```python
from build123d import *

# Parameters (mm, degrees)
CUT_EXTRUDE1_REACH  = 125.775
SKETCH2_R           = 3.3
SKETCH3_R           = 5.5
CUT_EXTRUDE2_DEPTH  = 6
CIRPATTERN1_COUNT   = 6
BOSS_EXTRUDE1_REACH = 125.775


with BuildPart() as part:
    # Sketch1 → Revolve1 (revolve)
    with BuildSketch(Plane.XY, mode=Mode.PRIVATE) as revolve1_sk:
        Polygon((-55.75, 38), (-43.75, 38), (-43.75, 25), (5, 25), (5, 23), (7, 23), (7, 25), (55.75, 25), (55.75, 16), (-55.75, 16), align=None)
    revolve(revolve1_sk.sketch.rotate(Axis((-82.106015927, 0, 0), (1, 0, 0)), 180), axis=Axis((-82.106015927, 0, 0), (1, 0, 0)))

    # Sketch2 → Cut-Extrude1 (cut, up to next)
    with BuildSketch(Plane.ZY.offset(55.75), mode=Mode.PRIVATE) as cut_extrude1_sk1:
        with Locations(Location((0, -31.5, 0), (0, 0, 270))):
            Circle(SKETCH2_R)
    cut_extrude1_tool1 = extrude(cut_extrude1_sk1.sketch, amount=-CUT_EXTRUDE1_REACH, mode=Mode.PRIVATE) & part.part
    cut_extrude1 = cut_extrude1_tool1.solids().sort_by_distance((-55.75, -31.5, 0))[0]
    add(cut_extrude1, mode=Mode.SUBTRACT)

    # Sketch3 → Cut-Extrude2 (cut)
    with BuildSketch(Plane.ZY.offset(55.75)):
        with Locations(Location((0, -31.5, 0), (0, 0, 270))):
            Circle(SKETCH3_R)
    cut_extrude2 = extrude(amount=-CUT_EXTRUDE2_DEPTH, mode=Mode.SUBTRACT)

    # CirPattern1: Cut-Extrude1, Cut-Extrude2 ×6 about axis, 1 skipped
    cirpattern1_axis = Axis((0, 0, 0), (-1, 0, 0))
    add([cut_extrude1.rotate(cirpattern1_axis, i * 360 / CIRPATTERN1_COUNT) for i in range(1, CIRPATTERN1_COUNT) if i not in (3,)], mode=Mode.SUBTRACT)
    add([cut_extrude2.rotate(cirpattern1_axis, i * 360 / CIRPATTERN1_COUNT) for i in range(1, CIRPATTERN1_COUNT) if i not in (3,)], mode=Mode.SUBTRACT)

    # Boss-Extrude1: up to this face of the body (flat: up to its plane)
    boss_extrude1_end = Plane(part.part.faces().sort_by_distance((-43.75, 36.925197693, 0))[0])
    # Sketch5 → Boss-Extrude1 (add, up to the picked face)
    with BuildSketch(Plane(origin=(55.75, 0, 0), x_dir=(0, 0, -1), z_dir=(1, 0, 0)), mode=Mode.PRIVATE) as boss_extrude1_sk1:
        with BuildLine():
            Line((-19, 30), (19, 30))
            Line((19, 30), (19, 16.248076809))
            ThreePointArc((19, 16.248076809), (0, 25), (-19, 16.248076809))
            Line((-19, 16.248076809), (-19, 30))
        make_face()
    boss_extrude1_tool1 = split(extrude(boss_extrude1_sk1.sketch, amount=-BOSS_EXTRUDE1_REACH, mode=Mode.PRIVATE), bisect_by=boss_extrude1_end, keep=Keep.BOTH, mode=Mode.PRIVATE)
    add(boss_extrude1_tool1.solids().sort_by(Axis((55.75, 25.748801, 0), (-1, 0, 0)))[0])


solid = part.part
```
Source: CAD feature listing. Evaluate the final solid. Frame: model axes, mm. A direction names the side the tool comes from. Round coordinates to 2 decimals unless told otherwise and drop trailing zeros. Loops run counter-clockwise (first coordinate to the right, second up) from the corner with the lowest first, then second, coordinate; pieces in that order, holes last. Notation, with made-up numbers: M 89,13.25 L 114,13.25 A16 ccw 114,20.25 Z; hole C -37.5,-31.5 d9. An arc over 180 degrees is marked long. Use a Markdown table: item, result. Add a question column.
1. Pull-direction query (Y, two-part tool) for faces 5 (the flat face through (-49.75, -17.5, 30.4)), 6 (the cylindrical face through (31.716, -24.987, 0.797)), 7 (the flat face through (-43.75, -25, -3)), 8 (the cylindrical face through (-53, -26, 0)); classes: +Y half, -Y half, draft (parallel to the pull), parting line (faces both ways), or undercut.
2. Cut plane B-B, the plane y = 0. Output: boundary loops of the cut face in (x, z), and give its area (3 significant figures).
3. Cut plane C-C, the plane x = -13. Output: boundary loops of the cut face in (y, z).
4. Cut plane A-A, the plane z = 0. Output: boundary loops of the cut face in (x, y).
5. Contact query for flat-ended pins moving along their axis: pin 1 (8 mm diameter, centred on x = -7, y = 5.5, fed in from -Z); pin 2 (9 mm diameter, centred on y = -31.5, z = 0, fed in from +X); pin 3 (15 mm diameter, centred on x = 7, y = 25.5, fed in from +Z). Output: stop coordinate, or through.
6. Cut plane D-D, the plane z = 12. Output: boundary loops of the cut face in (x, y).
7. Set-up query: faces 1 (the flat face through (7, 30, 0)), 2 (the cylindrical face through (6.014, 2.994, -22.804)), 3 (the cylindrical face through (-19.034, -24.987, 0.797)), 4 (the flat face through (-49.75, -15, -31)). Return all of +Z, -Z, +X, -X, +Y, -Y with unobstructed straight access to the full face (end or side cutting, diameter ignored); none if empty.
8. Ray query, line 1 along Z through (x, y) = (-48.1, -31.5); line 2 along Z through (x, y) = (-31, 0); line 3 along X through (y, z) = (17, 21). Return the intervals inside material, ascending. Write a range as [from, to].
Solution:
| question | item | result |
|---|---|---|
| 1 | face 5 | undercut |
| 1 | face 6 | parting line |
| 1 | face 7 | draft |
| 1 | face 8 | undercut |
| 2 | outline | M -55.75,-38 L -43.75,-38 L -43.75,-25 L 5,-25 L 5,-23 L 7,-23 L 7,-25 L 55.75,-25 L 55.75,-16 L -55.75,-16 Z; M -55.75,16 L 55.75,16 L 55.75,25 L 7,25 L 7,23 L 5,23 L 5,25 L -43.75,25 L -43.75,38 L -55.75,38 Z |
| 2 | area | 2,310 mm2 |
| 3 | outline | M 16.25,-19 L 30,-19 L 30,19 L 16.25,19 A25 ccw long Z; hole C 0,0 d32 |
| 4 | outline | M -55.75,-38 L -43.75,-38 L -43.75,-34.8 L -49.75,-34.8 L -49.75,-37 L -55.75,-37 Z; M -55.75,-26 L -49.75,-26 L -49.75,-28.2 L -43.75,-28.2 L -43.75,-25 L 5,-25 L 5,-23 L 7,-23 L 7,-25 L 55.75,-25 L 55.75,-16 L -55.75,-16 Z; M -55.75,16 L 55.75,16 L 55.75,30 L -43.75,30 L -43.75,38 L -55.75,38 Z; hole M 5,23 L 7,23 L 7,25 L 5,25 Z |
| 5 | pin 1 | stops at z = -24.95 |
| 5 | pin 2 | stops at x = -43.75 |
| 5 | pin 3 | stops at z = 19 |
| 6 | outline | M -55.75,-36.06 L -43.75,-36.06 L -43.75,-21.93 L 5,-21.93 L 5,-19.62 L 7,-19.62 L 7,-21.93 L 55.75,-21.93 L 55.75,-10.58 L -55.75,-10.58 Z; M -55.75,10.58 L 55.75,10.58 L 55.75,30 L -43.75,30 L -43.75,36.06 L -55.75,36.06 Z; hole M 5,19.62 L 7,19.62 L 7,21.93 L 5,21.93 Z |
| 7 | face 1 | +Z, -Z, +X, +Y |
| 7 | face 2 | none |
| 7 | face 3 | +X |
| 7 | face 4 | -X |
| 8 | line 1 | z = [-21.25, -3.3], [3.3, 21.25] |
| 8 | line 2 | z = [-25, -16], [16, 25] |
| 8 | line 3 | x = [-55.75, -43.75] |
